```python
from build123d import *

# Parameters (mm, degrees)
F1_DEPTH = 3
F3_DEPTH = 4
F4_R     = 1.5
F5_R     = 1


with BuildPart() as f1:
    # F0 (on Top) → F1 (new body, symmetric)
    with BuildSketch(Plane.XY):
        with BuildLine():
            Line((3, -40), (3, 0))
            ThreePointArc((3, 0), (2.1213203436, 2.1213203436), (0, 3))
            Line((0, 3), (-40, 3))
            ThreePointArc((-40, 3), (-42.1213203436, 2.1213203436), (-43, 0))
            Line((-43, 0), (-43, -16.2))
            ThreePointArc((-43, -16.2), (-42.1213203436, -18.3213203436), (-40, -19.2))
            Line((-40, -19.2), (-22.2, -19.2))
            ThreePointArc((-22.2, -19.2), (-20.0786796564, -20.0786796564), (-19.2, -22.2))
            Line((-19.2, -22.2), (-19.2, -40))
            ThreePointArc((-19.2, -40), (-18.3213203436, -42.1213203436), (-16.2, -43))
            Line((-16.2, -43), (0, -43))
            ThreePointArc((0, -43), (2.1213203436, -42.1213203436), (3, -40))
        make_face()
    extrude(amount=F1_DEPTH, both=True)

    # F2 (on Top) → F3 (cut)
    with BuildSketch(Plane.XY):
        Polygon((-16.2, 3), (-16.2, 0), (-43, 0), (-43, -16.2), (-16.2, -16.2), (-16.2, -43), (0, -43), (0, -16.2), (0, 0), (0, 3), align=None)
    extrude(amount=F3_DEPTH, mode=Mode.SUBTRACT)

    # F4
    f4_edges = [f1.edges().sort_by_distance(p)[0] for p in [
        (-18.32132, -42.12132, -3),
        (-8.1, -43, -3),
        (2.12132, -42.12132, -3),
        (3, -20, -3),
        (2.12132, 2.12132, -3),
        (-20, 3, -3),
        (-42.12132, 2.12132, -3),
        (-43, -8.1, -3),
        (-42.12132, -18.32132, -3),
        (-31.1, -19.2, -3),
        (-20.07868, -20.07868, -3),
        (-19.2, -31.1, -3),
    ]]
    fillet(f4_edges, radius=F4_R)

    # F5
    f5_edges = [f1.edges().sort_by_distance(p)[0] for p in [
        (-28.1, 3, 3),
        (-19.2, -31.1, 3),
        (-16.2, -16.2, 1.5),
    ]]
    fillet(f5_edges, radius=F5_R)


solid = f1.part
```
Source: CAD feature listing. Evaluate the final solid. Frame: model axes, mm. A direction names the side the tool comes from. Round coordinates to 2 decimals unless told otherwise and drop trailing zeros. Write each loop counter-clockwise with the first axis right and the second up, starting at its lowest first coordinate (ties: lowest second). Pieces come first, ordered by that corner, then holes. Notation, with made-up numbers: M 80,81.25 L 111,81.25 A24 ccw 111,103.25 Z; hole C -15.75,-22.5 d3. An arc over 180 degrees is marked long. Answer as a JSON object with one key per item and string values. Group by question number.
(1) First-contact query: pin 1 (2.5 mm diameter, centred on x = -33, z = 1, fed in from -Y); pin 2 (2.5 mm diameter, centred on y = -30.5, z = 2, fed in from -X); pin 3 (1.5 mm diameter, centred on y = 1, z = 1.5, fed in from +X). Flat tips, straight axial feed; report the tip coordinate or a pass-through.
(2) Section query A-A on z = 1. Output: boundary loops of the cut face in (x, y), then the cut area to 3 significant figures.
(3) Section query B-B on y = -4.5. Output: boundary loops of the cut face in (x, z).
(4) Mould query, pull axis X, two halves, no side actions, for faces 1 (the flat face through (-17, -15, 0)), 2 (the cylindrical face through (-7.99, -42.55, -2.57)), 3 (the flat face through (-19.2, -31, 0)). Classes: +X half, -X half, draft (parallel to the pull), parting line (faces both ways), or undercut.
(5) Section query C-C on x = -28.5. Output: boundary loops of the cut face in (y, z), then the cut area to 3 significant figures.
(6) Section query D-D on y = -36.5. Output: boundary loops of the cut face in (x, z).
(7) Ray query, line 1 (X direction, y = -27.5, z = 1.5); line 2 (Z direction, x = -16, y = -5). Return the intervals inside material, ascending. Write a range as [from, to].
(8) Reachability of faces 4 (the cylindrical face through (-30.98, -18.75, -2.57)), 5 (the flat face through (0, -20, 1)), 6 (the flat face through (-18, -23, 3)), 7 (the cylindrical face through (-18.915, -31.225, 2.699)), 8 (the flat face through (-29, 0, 1)) from +Z, -Z, +X, -X, +Y, -Y: full face, straight path, thin tool, end or side. Return the list, or none.
Computed values:
{
 "1": {"pin 1": "y = -19.2", "pin 2": "x = -19.2", "pin 3": "x = 2.99"},
 "2": {"outline": "M -43,-16.2 A3 ccw -40,-19.2 L -22.2,-19.2 A3 cw -19.2,-22.2 L -19.2,-40 A3 ccw -16.2,-43 L -16.2,-17.2 A1 ccw -17.2,-16.2 Z; M -43,0 L -16.2,0 L -16.2,3 L -40,3 A3 ccw Z; M 0,-43 A3 ccw 3,-40 L 3,0 A3 ccw 0,3 Z", "area": "362 mm^2"},
 "3": {"outline": "M -43,-1.5 A1.5 ccw -41.5,-3 L 1.5,-3 A1.5 ccw 3,-1.5 L 3,3 L 0,3 L 0,0 L -43,0 Z"},
 "4": {"face 1": "undercut", "face 2": "draft", "face 3": "-X half"},
 "5": {"outline": "M -19.2,-1.5 A1.5 ccw -17.7,-3 L 1.5,-3 A1.5 ccw 3,-1.5 L 3,2 A1 ccw 2,3 L 0,3 L 0,0 L -16.2,0 L -16.2,3 L -18.2,3 A1 ccw -19.2,2 Z", "area": "83.2 mm^2"},
 "6": {"outline": "M -19.2,-1.5 A1.5 ccw -17.7,-3 L 1.5,-3 A1.5 ccw 3,-1.5 L 3,3 L 0,3 L 0,0 L -16.2,0 L -16.2,3 L -18.2,3 A1 ccw -19.2,2 Z"},
 "7": {"line 1": "[-19.2, -16.2], [0, 3]", "line 2": "[-3, 0]"},
 "8": {"face 4": "-Z, -X, -Y", "face 5": "+Z, +Y, -Y", "face 6": "+Z, +X, -X, +Y, -Y", "face 7": "+Z, -X, -Y", "face 8": "+Z, -X"}
}
